Can you work these out from the drawing? Everything is in mm from the part's minimum corner. Give positions to 0.01 mm unless a question says otherwise; leave off trailing zeros. Order: outer loops, then holes, each group sorted by start corner. A loop starts at its lowest first (then second) coordinate and runs counter-clockwise, first axis right, second up. Notation, with made-up numbers: (72, 44) -> (80, 44) arc R29 cw to (80, 68) -> close; hole circle Ø10 at (85, -36.5). An arc over 180 degrees is marked (long way). Answer as CSV lines item,"result". Start each with the question number.
(1) I want a section at C-C (z = 12.25). Please give me the cut outline in (x, y).
(2) I need wall thicknesses on L1, parallel to Y at x = 30, z = 6.5; L2, parallel to Z at x = 10, y = 9.5. Which ranges of each line are inside material? Lowest first, please.
(3) I want a section at D-D (y = 19). Please give me the cut outline in (x, z).
(4) I want a section at A-A (y = 30). Please give me the cut outline in (x, z), plus the area to 3 significant figures.
(5) We'd pull the mould along X, two halves only. Please class the marked faces 1, 2 and 3: released by +X, released by -X, zero draft, split by the parting line, or undercut.
(6) Will these pins go through, and if not, where does the flat tip stop? pin 1 Ø6 at (x, z) = (18.5, 11) entering from -Y; pin 2 Ø3.5 at (x, y) = (32, 32) entering from +Z; pin 3 Ø2 at (x, z) = (25, 5) entering from -Y.
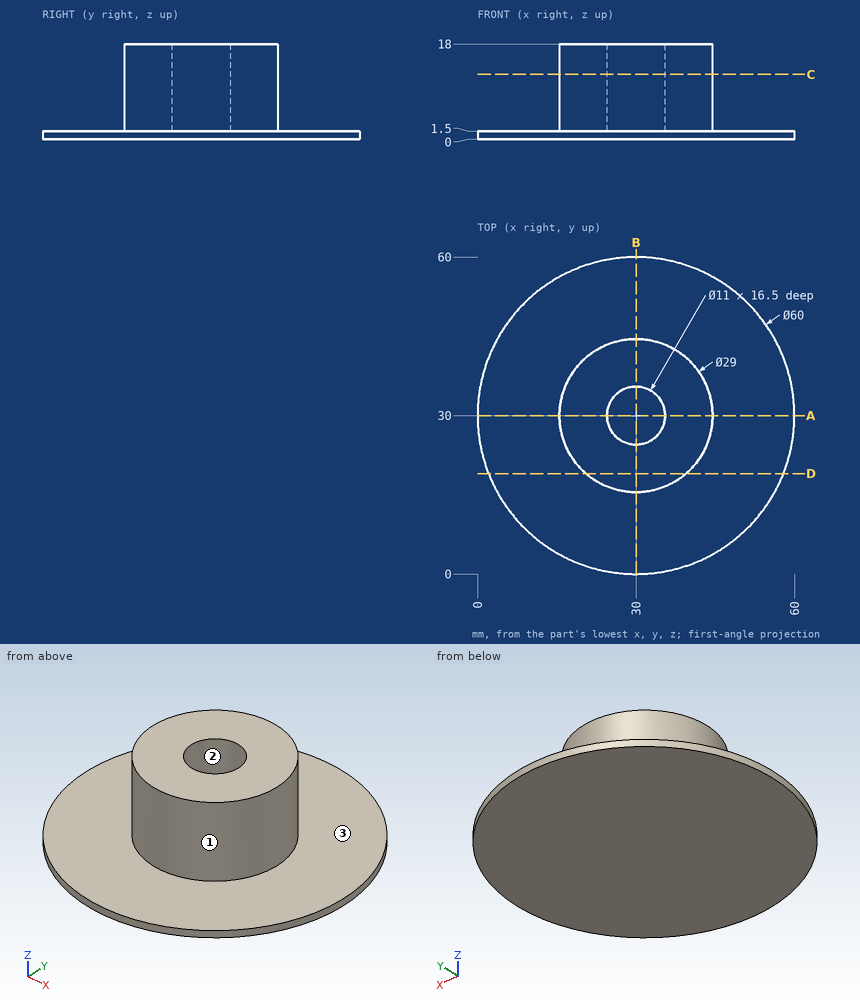
Final values:
1,outline,"circle Ø29 at (30, 30); hole circle Ø11 at (30, 30)"
2,L1,"15.5 to 24.5, 35.5 to 44.5"
2,L2,"0 to 1.5"
3,outline,"(2.09, 0) -> (57.91, 0) -> (57.91, 1.5) -> (39.45, 1.5) -> (39.45, 18) -> (20.55, 18) -> (20.55, 1.5) -> (2.09, 1.5) -> close"
4,outline,"(0, 0) -> (60, 0) -> (60, 1.5) -> (44.5, 1.5) -> (44.5, 18) -> (35.5, 18) -> (35.5, 1.5) -> (24.5, 1.5) -> (24.5, 18) -> (15.5, 18) -> (15.5, 1.5) -> (0, 1.5) -> close"
4,area,"387 mm²"
5,face 1,"split by the parting line"
5,face 2,"undercut"
5,face 3,"zero draft"
6,pin 1,"y = 18.25"
6,pin 2,"z = 1.5"
6,pin 3,"y = 16.06"
